Could you check a few things on this model? Use its own coordinates, in mm. Face numbers are marked on the shaded views. A direction names the side the tool comes from. Coordinates: 2 decimals unless noted, no trailing zeros. Write each loop counter-clockwise with the first axis right and the second up, starting at its lowest first coordinate (ties: lowest second). Pieces come first, ordered by that corner, then holes. Notation, with made-up numbers: (42, -21.5) - (76, -21.5) arc R14 ccw to (76, -13.5) - close; hole circle Ø7 at (79.25, -28.75). An arc over 180 degrees is marked (long way). Answer as a JSON object with one key per item and string values. Group by question number.
1) If we section it at A-A (z = 61.5): Write out the boundary of the cut face in (x, y).
2) If we section it at C-C (y = -24.5): Write out the boundary of the cut face in (x, z), plus the area to 3 significant figures.
3) On a 3-axis mill with a long thin cutter (end or side, diameter ignored), from which of +Z, -Z, +X, -X, +Y, -Y can I reach the whole of each face in a straight line? I mean the marked faces 4, 5 and 6. Say none if no direction works.
4) Will these pins go through, and if not, where does the flat tip stop? pin 1 Ø9.5 at (x, z) = (-9, -8.5) entering from +Y; pin 2 Ø24.5 at (y, z) = (-15, -6) entering from +X; pin 3 Ø4 at (y, z) = (-11, 6.5) entering from +X.
5) If we section it at D-D (x = -57.5): Write out the boundary of the cut face in (y, z), plus the area to 3 significant figures.
6) If we section it at B-B (x = -17.5): Write out the boundary of the cut face in (y, z), plus the area to 3 significant figures.
7) Please list where these lines run through material, in increasing order: line 1 along X through (y, z) = (-10, 71); line 2 along X through (y, z) = (-39.5, -11); line 3 along Z through (x, y) = (-10.5, -72).
8) We'd pull the mould along X, two halves only. Please class the marked faces 1, 2 and 3: released by +X, released by -X, zero draft, split by the parting line, or undercut.
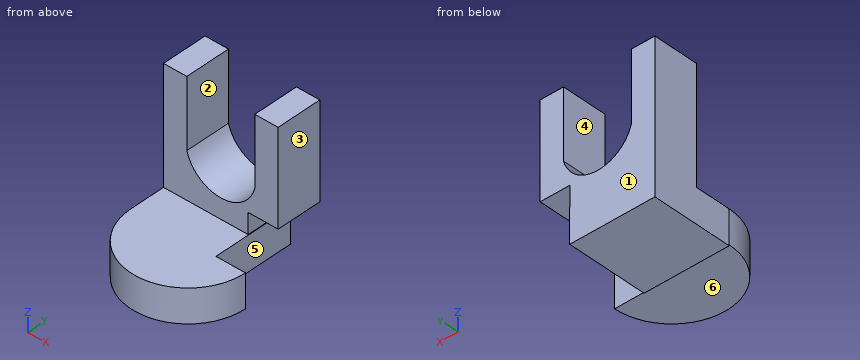
```python
from build123d import *

# Parameters (mm, degrees)
F1_DEPTH = 29.718
F0_W     = 75.3477662802
F0_H     = 22.4088169634
F2_DEPTH = 53.086
F4_DEPTH = 21.844
F5_W     = 19.3952620029
F5_H     = 23.368
F6_DEPTH = 22.4098169634
F8_DEPTH = 29.719


with BuildPart() as f1:
    # F0 (on Front) → F1 (new body)
    with BuildSketch(Plane.XZ):
        with BuildLine():
            Line((-60.0075013936, 75.3477662802), (-75.3477662802, 75.3477662802))
            Line((-75.3477662802, 75.3477662802), (-75.3477662802, 0))
            Line((-75.3477662802, 0), (0, 0))
            Line((0, 0), (0, 75.3477662802))
            Line((0, 75.3477662802), (-15.3402648866, 75.3477662802))
            Line((-15.3402648866, 75.3477662802), (-15.3402648866, 30.2293412387))
            ThreePointArc((-15.3402648866, 30.2293412387), (-37.6738831401, 13.0326763907), (-60.0075013936, 30.2293412387))
            Line((-60.0075013936, 30.2293412387), (-60.0075013936, 75.3477662802))
        make_face()
    extrude(amount=F1_DEPTH)

    # F0 (on Front) → F2 (join)
    with BuildSketch(Plane.XZ):
        with Locations((-37.6738831401, -11.2044084817)):
            Rectangle(F0_W, F0_H)
    extrude(amount=F2_DEPTH)

    # F3 (on face) → F4 (join)
    with BuildSketch(Plane.XY):
        with BuildLine():
            Line((0, -53.086), (-75.3477662802, -53.086))
            ThreePointArc((-75.3477662802, -53.086), (-37.6738831401, -90.7598831401), (0, -53.086))
        make_face()
    extrude(amount=-F4_DEPTH)

    # F5 (on face) → F6 (cut, through all)
    with BuildSketch(Plane.XY):
        with Locations((-9.6976310015, -41.402)):
            Rectangle(F5_W, F5_H)
    extrude(amount=-F6_DEPTH, mode=Mode.SUBTRACT)

    # F7 (on face) → F8 (cut, through all)
    with BuildSketch(Plane.XZ.offset(29.718)):
        Polygon((0, 13.4468190372), (-19.6963120252, 13.4468190372), (-19.6963120252, 0), (-19.3952620029, 0), (-19.3952620029, -22.4088169634), (0, -22.4088169634), align=None)
    extrude(amount=-F8_DEPTH, mode=Mode.SUBTRACT)


solid = f1.part
```
Here are the results:
{
 "1": {"outline": "(-75.35, -29.72) - (-60.01, -29.72) - (-60.01, 0) - (-75.35, 0) - close; (-15.34, -29.72) - (0, -29.72) - (0, 0) - (-15.34, 0) - close"},
 "2": {"outline": "(-75.35, -22.41) - (-19.4, -22.41) - (-19.4, 0) - (-19.7, 0) - (-19.7, 13.45) - (0, 13.45) - (0, 75.35) - (-15.34, 75.35) - (-15.34, 30.23) arc R23.1 cw to (-60.01, 30.23) - (-60.01, 75.35) - (-75.35, 75.35) - close", "area": "4,080 mm²"},
 "3": {"face 4": "+Z, +Y, -Y", "face 5": "-Z, +X, +Y", "face 6": "-Z, +X, -X, -Y"},
 "4": {"pin 1": "stops at y = -53.09", "pin 2": "stops at x = -19.4", "pin 3": "stops at x = -19.7"},
 "5": {"outline": "(-85.12, -21.84) - (-53.09, -21.84) - (-53.09, -22.41) - (0, -22.41) - (0, 24.28) - (-29.72, 24.28) - (-29.72, 0) - (-85.12, 0) - close", "area": "2,610 mm²"},
 "6": {"outline": "(-84.9, -21.84) - (-53.09, -21.84) - (-53.09, 0) - (-84.9, 0) - close; (-29.72, 13.45) - (0, 13.45) - (0, 24.88) - (-29.72, 24.88) - close", "area": "1,030 mm²"},
 "7": {"line 1": "x = -75.35 to -60.01, -15.34 to 0", "line 2": "x = -75.35 to -19.4", "line 3": "z = -21.84 to 0"},
 "8": {"face 1": "zero draft", "face 2": "undercut", "face 3": "released by +X"}
}
